Part model, mm, in its own coordinate system. Give positions to 0.01 mm unless a question says otherwise; leave off trailing zeros. Loops run counter-clockwise (first coordinate to the right, second up) from the corner with the lowest first, then second, coordinate; pieces in that order, holes last. Notation, with made-up numbers: M 12.25,33.25 L 23.25,33.25 A22 ccw 23.25,43.25 Z; hole C 31,-8 d3. An arc over 180 degrees is marked long. Answer in a Markdown table with one row per item.
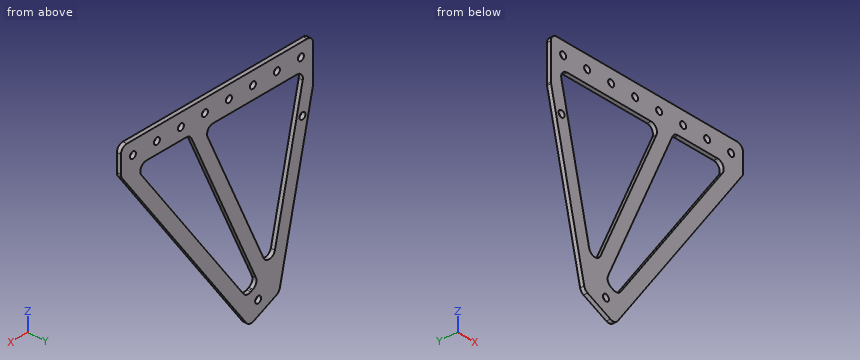
from build123d import *

# Parameters (mm, degrees)
SKETCH1_R           = 2
BOSS_EXTRUDE1_DEPTH = 2.5
FILLET2_R           = 4


with BuildPart() as part:
    # Sketch1 → Boss-Extrude1 (new body)
    with BuildSketch(Plane(origin=(0, 0, 0), x_dir=(1, 0, 0), z_dir=(0, 1, 0))):
        Polygon((-24, -8), (24, -8), (24, 8), (-61.475760907, 128.370940703), (-81.524239093, 119.312324779), (-104.126855641, 18.58956294), (-104.126855641, -8), (-86.093666761, -8), align=None)
        with Locations(Location((-16, 0, 0), (0, 0, 270))):
            Circle(SKETCH1_R, mode=Mode.SUBTRACT)
        with Locations(Location((16, 0, 0), (0, 0, 270))):
            Circle(SKETCH1_R, mode=Mode.SUBTRACT)
        with Locations(Location((0, 0, 0), (0, 0, 270))):
            Circle(SKETCH1_R, mode=Mode.SUBTRACT)
        with Locations(Location((-67.5, 116.913429511, 0), (0, 0, 270))):
            Circle(SKETCH1_R, mode=Mode.SUBTRACT)
        with Locations(Location((-32, 0, 0), (0, 0, 270))):
            Circle(SKETCH1_R, mode=Mode.SUBTRACT)
        with Locations(Location((-48, 0, 0), (0, 0, 270))):
            Circle(SKETCH1_R, mode=Mode.SUBTRACT)
        with Locations(Location((-64, 0, 0), (0, 0, 270))):
            Circle(SKETCH1_R, mode=Mode.SUBTRACT)
        with Locations(Location((-80, 0, 0), (0, 0, 270))):
            Circle(SKETCH1_R, mode=Mode.SUBTRACT)
        with Locations(Location((-96, 0, 0), (0, 0, 270))):
            Circle(SKETCH1_R, mode=Mode.SUBTRACT)
        with Locations(Location((-97.021679837, 31.983686003, 0), (0, 0, 270))):
            Circle(SKETCH1_R, mode=Mode.SUBTRACT)
        Polygon((-31.229369404, 8), (-76.046035256, 107.187994635), (-98.304243511, 8), align=None, mode=Mode.SUBTRACT)
        Polygon((-63.480229926, 109.950983508), (-59.488316608, 111.754672009), (14.80532848, 7.130906714), (-22.057960952, 7.130906714), (-67.661999872, 108.061511027), align=None, mode=Mode.SUBTRACT)
    extrude(amount=BOSS_EXTRUDE1_DEPTH)

    # Fillet2
    fillet2_edges = [part.edges().sort_by_distance(p)[0] for p in [
        (24, 1.25, -8),
        (24, 1.25, 8),
        (-104.126855641, 1.25, 8),
        (-104.126855641, 1.25, -18.58956294),
        (-81.524239093, 1.25, -119.312324779),
        (-61.475760907, 1.25, -128.370940703),
        (-67.661999872, 1.25, -108.061511027),
        (-22.057960952, 1.25, -7.130906714),
        (14.80532848, 1.25, -7.130906714),
        (-59.488316608, 1.25, -111.754672009),
        (-98.304243511, 1.25, -8),
        (-31.229369404, 1.25, -8),
        (-76.046035256, 1.25, -107.187994635),
    ]]
    fillet(fillet2_edges, radius=FILLET2_R)


solid = part.part
(1) Drill centre lines: line 1 along X through (y, z) = (1.7, -69.5); line 2 along X through (y, z) = (2.2, -83.5); line 3 along Z through (x, y) = (-62.5, 0.95). Where is each one in solid material? Low to high.
Recorded:
| item | result |
|---|---|
| line 1 | x = -92.7 to -84.5, -59.02 to -50.24, -29.48 to -19.67 |
| line 2 | x = -89.56 to -81.36, -65.34 to -56.56, -39.42 to -29.61 |
| line 3 | z = -127.36 to -110.39, -96.64 to -77.21, -8 to -1.32, 1.32 to 8 |
(2) Saw through at D-D (x = 16). Write the cut outline in (y, z), plus the area to 3 significant figures.
Recorded:
| item | result |
|---|---|
| outline | M 0,-19.27 L 2.5,-19.27 L 2.5,-2 L 0,-2 Z; M 0,2 L 2.5,2 L 2.5,8 L 0,8 Z |
| area | 58.2 mm^2 |
(3) Saw through at A-A (x = -5.5). Write the cut outline in (y, z).
Recorded:
| item | result |
|---|---|
| outline | M 0,-49.54 L 2.5,-49.54 L 2.5,-35.73 L 0,-35.73 Z; M 0,-7.13 L 2.5,-7.13 L 2.5,8 L 0,8 Z |
(4) Saw through at C-C (z = 0). Give the number of separate pieces and of enclosed holes in the cut face, plus the area to 3 significant figures.
Recorded:
| item | result |
|---|---|
| separate pieces | 9 |
| enclosed holes | 0 |
| area | 240 mm^2 |
(5) Pin check, flat tips, straight feed: pin 1 Ø1.5 at (y, z) = (1.5, -51) entering from -X; pin 2 Ø1.2 at (x, y) = (-58.5, 0.5) entering from -Z; pin 3 Ø0.8 at (x, y) = (-10.5, 1.5) entering from -Z. Stop position of each tip, or through.
Recorded:
| item | result |
|---|---|
| pin 1 | stops at x = -97.02 |
| pin 2 | stops at z = -125.03 |
| pin 3 | stops at z = -57.15 |
(6) Saw through at B-B (z = -84). Write the cut outline in (x, y), plus the area to 3 significant figures.
Recorded:
| item | result |
|---|---|
| outline | M -89.45,0 L -81.25,0 L -81.25,2.5 L -89.45,2.5 Z; M -65.57,0 L -56.79,0 L -56.79,2.5 L -65.57,2.5 Z; M -39.78,0 L -29.97,0 L -29.97,2.5 L -39.78,2.5 Z |
| area | 67.0 mm^2 |
